CAD build for the part. Positions are in the model's coordinates, mm. Face numbers are marked on the shaded views. A direction names the side the tool comes from. Round coordinates to 2 decimals unless told otherwise and drop trailing zeros. Order: outer loops, then holes, each group sorted by start corner. A loop starts at its lowest first (then second) coordinate and runs counter-clockwise, first axis right, second up. Notation, with made-up numbers: (38, -13) -> (45, -13) arc R3 cw to (45, -9) -> close; hole circle Ø1 at (34, 78.25). An arc over 180 degrees is marked (long way). Return JSON: item names as keys, results as strings. Group by question number.
Q1. Cut at D-D (x = -15). Write the cut outline in (y, z), then the cut area to 3 significant figures.
Q2. Mould opens along Y. For the marked faces 5, 6 and 7 say: +Y half, -Y half, draft (parallel to the pull), parting line (faces both ways), or undercut.
Q3. Cut at C-C (y = 9.5). Write the cut outline in (x, z).
Q4. Flat gauge pins, fed straight in: pin 1 (4 mm diameter, centred on x = 10, z = -4.5, fed in from -Y); pin 2 (4 mm diameter, centred on x = 17.5, y = 9.9, fed in from +Z); pin 3 (8 mm diameter, centred on x = 7, y = 4, fed in from -Z); pin 4 (6 mm diameter, centred on x = 8, z = 3.5, fed in from +Y). Where does each tip first touch, or does it go through?
Q5. Probe line 1 along X through (y, z) = (2.05, 0); line 2 along X through (y, z) = (5.25, -5); line 3 along Y through (x, z) = (-17.5, -4.5). List the from-to ranges inside material, lowest first.
Q6. Cut at A-A (z = -2.75). Write the cut outline in (x, y), then the cut area to 3 significant figures.
Q7. Which spindle directions (+Z, -Z, +X, -X, +Y, -Y) get a long thin tool onto all of the face, cutting with end or side? Do the marked faces 1, 2, 3 and 4. Say none if no direction does.
Q8. Cut at B-B (z = 0). Write the cut outline in (x, y), then the cut area to 3 significant figures.
from build123d import *

# Parameters (mm, degrees)
SKETCH1_R           = 1.1
BOSS_EXTRUDE1_DEPTH = 3
FILLET1_R           = 3
SKETCH2_R           = 1.6
BOSS_EXTRUDE2_DEPTH = 3
FILLET2_R           = 5
FILLET3_R           = 3


with BuildPart() as part:
    # Sketch1 → Boss-Extrude1 (new body)
    with BuildSketch(Plane(origin=(0, 0, 0), x_dir=(1, 0, 0), z_dir=(0, 1, 0))):
        Polygon((-16.9, -9.2), (16.9, -9.2), (16.9, 6.2), (11.4, 6.2), (11.4, -6.2), (-11.4, -6.2), (-11.4, 6.2), (-16.9, 6.2), align=None)
        with Locations(Location((-14.35, 0, 0), (0, 0, 270))):
            Circle(SKETCH1_R, mode=Mode.SUBTRACT)
        with Locations(Location((14.35, 0, 0), (0, 0, 270))):
            Circle(SKETCH1_R, mode=Mode.SUBTRACT)
    extrude(amount=BOSS_EXTRUDE1_DEPTH)

    # Fillet1
    fillet1_edges = [part.edges().sort_by_distance(p)[0] for p in [
        (16.9, 1.5, 9.2),
        (-16.9, 1.5, 9.2),
    ]]
    fillet(fillet1_edges, radius=FILLET1_R)

    # Sketch2 → Boss-Extrude2 (add)
    # profile 1 of 2: a face of its own
    with BuildSketch(Plane(origin=(0, 0, -6.2), x_dir=(-1, 0, 0), z_dir=(0, 0, -1))):
        Polygon((-16.35, 3), (-16.35, 5.7), (-12.5, 10.288251331), (-12.5, 14.9), (-22.5, 14.9), (-22.5, 4.9), (-22.5, 0), (-16.9, 0), (-16.9, 3), align=None)
        with Locations((-17.5, 9.9)):
            Circle(SKETCH2_R, mode=Mode.SUBTRACT)
    # profile 2 of 2: a face of its own
    with BuildSketch(Plane(origin=(0, 0, -6.2), x_dir=(-1, 0, 0), z_dir=(0, 0, -1))):
        Polygon((22.5, 14.9), (22.5, 4.9), (22.5, 0), (16.9, 0), (16.9, 3), (16.35, 3), (16.35, 5.7), (12.5, 10.288251331), (12.5, 14.9), align=None)
        with Locations((17.5, 9.9)):
            Circle(SKETCH2_R, mode=Mode.SUBTRACT)
    extrude(amount=-BOSS_EXTRUDE2_DEPTH)

    # Fillet2
    # the kernel refuses this fillet: 5 mm, written as the material it takes off along each edge
    with BuildSketch(Plane(origin=(22.5, 0, -18.7), x_dir=(0, 1, 0), z_dir=(0, 0, 1)), Plane(origin=(-22.5, 14.9, -18.7), x_dir=(0, -1, 0), z_dir=(0, 0, 1))) as fillet2_piece_1:
        with BuildLine():
            CenterArc((FILLET2_R, FILLET2_R), FILLET2_R, 180, 90)
            Line((0, FILLET2_R), (-FILLET2_R * 0.02, FILLET2_R))
            Line((-FILLET2_R * 0.02, FILLET2_R), (-FILLET2_R * 0.02, -FILLET2_R * 0.02))
            Line((-FILLET2_R * 0.02, -FILLET2_R * 0.02), (FILLET2_R, -FILLET2_R * 0.02))
            Line((FILLET2_R, -FILLET2_R * 0.02), (FILLET2_R, 0))
        make_face()
    extrude(amount=28, mode=Mode.SUBTRACT)
    with BuildSketch(Plane(origin=(-22.5, 0, -18.7), x_dir=(0, 1, 0), z_dir=(0, 0, 1)), Plane(origin=(22.5, 14.9, -18.7), x_dir=(0, -1, 0), z_dir=(0, 0, 1))) as fillet2_piece_2:
        with BuildLine():
            CenterArc((FILLET2_R, -FILLET2_R), FILLET2_R, 90, 90)
            Line((0, -FILLET2_R), (-FILLET2_R * 0.02, -FILLET2_R))
            Line((-FILLET2_R * 0.02, -FILLET2_R), (-FILLET2_R * 0.02, FILLET2_R * 0.02))
            Line((-FILLET2_R * 0.02, FILLET2_R * 0.02), (FILLET2_R, FILLET2_R * 0.02))
            Line((FILLET2_R, FILLET2_R * 0.02), (FILLET2_R, 0))
        make_face()
    extrude(amount=28, mode=Mode.SUBTRACT)
    with BuildSketch(Plane(origin=(-12.5, 14.9, -18.662258248), x_dir=(-1, 0, 0), z_dir=(0, 0, 1))) as fillet2_piece_3:
        with BuildLine():
            CenterArc((4.984903299, 5), FILLET2_R, 184.453515666, 85.546484334)
            Line((0, 4.611748669), (-0.099698066, 4.603983642))
            ThreePointArc((-0.099698066, 4.603983642), (-0.1, 2.305874334), (-0.1, 0))
            Line((-0.1, 0), (0, -0.1))
            Line((0, -0.1), (4.984903299, -0.1))
            Line((4.984903299, -0.1), (4.984903299, 0))
        make_face()
    extrude(amount=27.924516497, mode=Mode.SUBTRACT)
    with BuildSketch(Plane(origin=(12.5, 14.9, -18.662258248), x_dir=(1, 0, 0), z_dir=(0, 0, 1))) as fillet2_piece_4:
        with BuildLine():
            CenterArc((4.984903299, -5), FILLET2_R, 90, 85.546484334)
            Line((0, -4.611748669), (-0.099698066, -4.603983642))
            ThreePointArc((-0.099698066, -4.603983642), (-0.1, -2.305874334), (-0.1, 0))
            Line((-0.1, 0), (0, 0.1))
            Line((0, 0.1), (4.984903299, 0.1))
            Line((4.984903299, 0.1), (4.984903299, 0))
        make_face()
    extrude(amount=27.924516497, mode=Mode.SUBTRACT)

    # Fillet3
    fillet3_edges = [part.edges().sort_by_distance(p)[0] for p in [
        (-12.5, 10.288251331, -4.7),
        (12.5, 10.288251331, -4.7),
    ]]
    fillet(fillet3_edges, radius=FILLET3_R)


solid = part.part
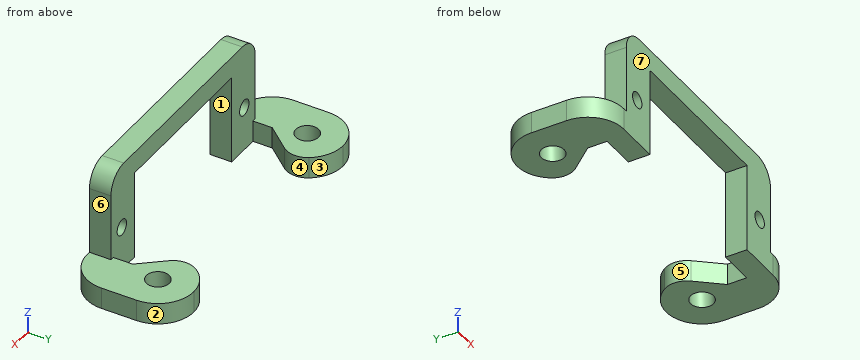
Solution:
{
 "1": {"outline": "(0, -6.2) -> (3, -6.2) -> (3, -0.89) -> (0, -0.89) -> close; (0, 0.89) -> (3, 0.89) -> (3, 8.99) -> (0, 8.99) -> close; (7.31, -6.2) -> (14.24, -6.2) -> (14.24, -3.2) -> (7.31, -3.2) -> close", "area": "61.0 mm²"},
 "2": {"face 5": "undercut", "face 6": "draft", "face 7": "-Y half"},
 "3": {"outline": "(-22.5, -6.2) -> (-19.05, -6.2) -> (-19.05, -3.2) -> (-22.5, -3.2) -> close; (-15.95, -6.2) -> (-13.22, -6.2) -> (-13.22, -3.2) -> (-15.95, -3.2) -> close; (13.22, -6.2) -> (15.95, -6.2) -> (15.95, -3.2) -> (13.22, -3.2) -> close; (19.05, -6.2) -> (22.5, -6.2) -> (22.5, -3.2) -> (19.05, -3.2) -> close"},
 "4": {"pin 1": "stops at y = 0", "pin 2": "stops at z = -3.2", "pin 3": "stops at z = 6.2", "pin 4": "stops at y = 3"},
 "5": {"line 1": "x = -16.9 to -15.45, -13.25 to -11.4, 11.4 to 13.25, 15.45 to 16.9", "line 2": "x = -22.5 to -16.35, 16.35 to 22.5", "line 3": "y = 0 to 8.3, 11.5 to 14.9"},
 "6": {"outline": "(-16.9, 0) -> (-11.4, 0) -> (-11.4, 3) -> (-16.9, 3) -> close; (11.4, 0) -> (16.9, 0) -> (16.9, 3) -> (11.4, 3) -> close", "area": "33.0 mm²"},
 "7": {"face 1": "-Z, +Y, -Y", "face 2": "+Z, -Z, +X, +Y", "face 3": "+Z, -Z, +Y", "face 4": "+Z, -Z"},
 "8": {"outline": "(-16.9, 0) -> (-15.45, 0) -> (-15.45, 3) -> (-16.9, 3) -> close; (-13.25, 0) -> (-11.4, 0) -> (-11.4, 3) -> (-13.25, 3) -> close; (11.4, 0) -> (13.25, 0) -> (13.25, 3) -> (11.4, 3) -> close; (15.45, 0) -> (16.9, 0) -> (16.9, 3) -> (15.45, 3) -> close", "area": "19.8 mm²"}
}
